Read the model definition and answer for the solid it produces. Units are mm, in the model's axes. A direction names the side the tool comes from. Give positions to 0.01 mm unless a question says otherwise; leave off trailing zeros. Loops run counter-clockwise (first coordinate to the right, second up) from the corner with the lowest first, then second, coordinate; pieces in that order, holes last. Notation, with made-up numbers: (35, 15) -> (93, 15) arc R16 cw to (93, 22) -> close; hole circle Ø3 at (33, 23.25). An arc over 180 degrees is marked (long way). One line per item, written item: value. Start each with the question number.
from build123d import *

# Parameters (mm, degrees)
EXTRUDE_1_DEPTH     = 6
SKETCH_2_R          = 1.65
CUT_EXTRUDE_1_DEPTH = 8


with BuildPart() as part:
    # 草图1 → 凸台-拉伸1 (new body)
    with BuildSketch(Plane(origin=(0, 0, 0), x_dir=(1, 0, 0), z_dir=(0, 1, 0))):
        Polygon((-11.5, 0.5), (-11.5, 6), (-10.5, 7), (10.5, 7), (11.5, 6), (11.5, 0.5), (4.5, 0.5), (4.5, 2.75), (3.5, 3.75), (-3.5, 3.75), (-4.5, 2.75), (-4.5, 0.5), align=None)
    extrude(amount=EXTRUDE_1_DEPTH)

    # 草图2 → 切除-拉伸1 (cut)
    with BuildSketch(Plane.XY.offset(-0.5)):
        with Locations((-7.5, 3)):
            Circle(SKETCH_2_R)
        with Locations((7.5, 3)):
            Circle(SKETCH_2_R)
    extrude(amount=-CUT_EXTRUDE_1_DEPTH, mode=Mode.SUBTRACT)


solid = part.part
Item 1: Section A-A, the plane z = -1.25 is taken. Determine the outline of the cut face in (x, y), plus the area to 3 significant figures.
Item 2: Section D-D, the plane z = -4 is taken. Determine the outline of the cut face in (x, y).
Item 3: Flat-ended cylindrical pins translate along their axes: pin 1 (3 mm diameter, centred on x = 1, y = 4, fed in from +Z); pin 2 (1.5 mm diameter, centred on x = -9, y = 3.5, fed in from -Z). Find the tip coordinate at first contact, or state that the pin passes through.
Item 4: Section B-B, the plane y = 3 is taken. Determine the outline of the cut face in (x, z).
Item 5: Consider L1, parallel to X at y = 3.1, z = -5.75; L2, parallel to X at y = 5.05, z = -2.5; L3, parallel to X at y = 4.5, z = -2.5. Determine where each line is inside the solid, lowest interval first. Write a range as [from, to].
Item 6: Section C-C, the plane x = -7.5 is taken. Determine the outline of the cut face in (y, z).
Item 7: Determine the mould class of faces 3 (the flat face through (0, 6, -4)), 4 (the flat face through (11.5, 3, -3)), 5 (the cylindrical face through (6.284, 4.115, -3.704)) for opening direction Y: pulls with the +Y half, pulls with the -Y half, needs draft (parallel to the pull), parting line crosses it, or undercut.
Item 8: For faces 1 (the flat face through (-3.99, 2.96, -3.26)), 2 (the flat face through (0, 3, -7)), determine the directions among +Z, -Z, +X, -X, +Y, -Y from which every point of the face is accessible in a straight line to the end or side of a thin tool.
Computed values:
1. outline: (-11.5, 0) -> (-4.5, 0) -> (-4.5, 6) -> (-11.5, 6) -> close; (4.5, 0) -> (11.5, 0) -> (11.5, 6) -> (4.5, 6) -> close; hole circle Ø3.3 at (-7.5, 3); hole circle Ø3.3 at (7.5, 3)
1. area: 66.9 mm²
2. outline: (-11.5, 0) -> (11.5, 0) -> (11.5, 6) -> (-11.5, 6) -> close; hole circle Ø3.3 at (-7.5, 3); hole circle Ø3.3 at (7.5, 3)
3. pin 1: z = -3.75
3. pin 2: z = -7
4. outline: (-11.5, -6) -> (-10.5, -7) -> (-9.15, -7) -> (-9.15, -0.5) -> (-11.5, -0.5) -> close; (-5.85, -7) -> (5.85, -7) -> (5.85, -0.5) -> (4.5, -0.5) -> (4.5, -2.75) -> (3.5, -3.75) -> (-3.5, -3.75) -> (-4.5, -2.75) -> (-4.5, -0.5) -> (-5.85, -0.5) -> close; (9.15, -7) -> (10.5, -7) -> (11.5, -6) -> (11.5, -0.5) -> (9.15, -0.5) -> close
5. L1: [-11.5, -9.15], [-5.85, 5.85], [9.15, 11.5]
5. L2: [-11.5, -4.5], [4.5, 11.5]
5. L3: [-11.5, -8.19], [-6.81, -4.5], [4.5, 6.81], [8.19, 11.5]
6. outline: (0, -7) -> (1.35, -7) -> (1.35, -0.5) -> (0, -0.5) -> close; (4.65, -7) -> (6, -7) -> (6, -0.5) -> (4.65, -0.5) -> close
7. face 3: pulls with the +Y half
7. face 4: needs draft
7. face 5: undercut
8. face 1: +Z, +Y, -Y
8. face 2: -Z, +X, -X, +Y, -Y
